from build123d import *

# Parameters (mm, degrees)
ESBO_O1_R                = 3.5
RESSALTO_EXTRUS_O1_DEPTH = 6
FILETE1_R                = 3
CHANFRO1_SIZE            = 2
CORTE_EXTRUS_O1_DEPTH    = 6
RESSALTO_EXTRUS_O2_DEPTH = 6
CORTE_EXTRUS_O2_DEPTH    = 10
FILETE2_R                = 2
CORTE_EXTRUS_O3_DEPTH    = 10
CORTE_EXTRUS_O4_DEPTH    = 201.089979759
CORTE_EXTRUS_O5_DEPTH    = 201.089979759
FILETE3_R                = 3


with BuildPart() as part:
    # Esboço1 → Ressalto-extrusão1 (new body)
    with BuildSketch(Plane.XY):
        with BuildLine():
            Line((23.094010768, 160), (88, 160))
            Line((88, 160), (100, 142.530265141))
            Line((100, 142.530265141), (100, 114))
            Line((100, 114), (84, 114))
            Line((84, 114), (69, 135.837168574))
            Line((69, 135.837168574), (69, 144))
            ThreePointArc((69, 144), (65, 148), (61, 144))
            Line((61, 144), (61, 135.837168574))
            Line((61, 135.837168574), (38, 96))
            Line((38, 96), (38, 0))
            Line((38, 0), (0, 0))
            Line((0, 0), (0, 120))
            Line((0, 120), (23.094010768, 160))
        make_face()
        with Locations((19, 12)):
            Circle(ESBO_O1_R, mode=Mode.SUBTRACT)
        with Locations((19, 24)):
            Circle(ESBO_O1_R, mode=Mode.SUBTRACT)
        with Locations((19, 36)):
            Circle(ESBO_O1_R, mode=Mode.SUBTRACT)
        with Locations((92, 122)):
            Circle(ESBO_O1_R, mode=Mode.SUBTRACT)
        with Locations((38, 122)):
            Circle(ESBO_O1_R, mode=Mode.SUBTRACT)
        with BuildLine():
            Line((41, 156), (49, 156))
            ThreePointArc((49, 156), (51, 154), (49, 152))
            Line((49, 152), (41, 152))
            ThreePointArc((41, 152), (39, 154), (41, 156))
        make_face(mode=Mode.SUBTRACT)
        with BuildLine():
            Line((8, 115), (8, 105))
            ThreePointArc((8, 105), (6, 103), (4, 105))
            Line((4, 105), (4, 115))
            ThreePointArc((4, 115), (6, 117), (8, 115))
        make_face(mode=Mode.SUBTRACT)
    extrude(amount=RESSALTO_EXTRUS_O1_DEPTH)

    # Filete1
    filete1_edges = [part.edges().sort_by_distance(p)[0] for p in [
        (100, 114, 3),
        (84, 114, 3),
        (69, 135.837168574, 3),
        (61, 135.837168574, 3),
        (38, 96, 3),
    ]]
    fillet(filete1_edges, radius=FILETE1_R)

    # Chanfro1
    chanfro1_edges = [part.edges().sort_by_distance(p)[0] for p in [
        (38, 0, 3),
        (0, 0, 3),
    ]]
    chamfer(chanfro1_edges, length=CHANFRO1_SIZE)

    # Esboço2 → Corte-extrusão1 (cut)
    with BuildSketch(Plane.XY.offset(6)):
        with BuildLine():
            Line((75, 152), (75, 141.231728845))
            Line((75, 141.231728845), (85.255212875, 126.30207469))
            ThreePointArc((85.255212875, 126.30207469), (88.154001919, 129.014862704), (92, 130))
            Line((92, 130), (92, 140.047327347))
            Line((92, 140.047327347), (83.789682385, 152))
            Line((83.789682385, 152), (75, 152))
        make_face()
        with BuildLine():
            Line((38, 130), (38, 140.047327347))
            Line((38, 140.047327347), (40.28207662, 144))
            Line((40.28207662, 144), (55, 144))
            Line((55, 144), (55, 141.444863729))
            Line((55, 141.444863729), (45.452626018, 124.908326913))
            ThreePointArc((45.452626018, 124.908326913), (42.512947191, 128.605551275), (38, 130))
        make_face()
    extrude(amount=-CORTE_EXTRUS_O1_DEPTH, mode=Mode.SUBTRACT)

    # Esboço3 → Ressalto-extrusão2 (add, through all)
    with BuildSketch(Plane.XY.offset(6)):
        Polygon((100, 142.530265141), (120, 113.414040375), (120, 77), (117, 74), (102.060706719, 74), (100, 77), (100, 90.707020188), (83.106053471, 115.301417403), (100, 117), align=None)
    extrude(amount=-RESSALTO_EXTRUS_O2_DEPTH)

    # Esboço4 → Corte-extrusão2 (cut)
    with BuildSketch(Plane.XY.offset(6)):
        with BuildLine():
            Line((105.122276139, 120.943770271), (114, 108.019480105))
            Line((114, 108.019480105), (114, 80))
            Line((114, 80), (106, 80))
            Line((106, 80), (106, 96.101580458))
            Line((106, 96.101580458), (93.595183818, 114.160651265))
            ThreePointArc((93.595183818, 114.160651265), (97.506753293, 116.196925973), (99.745062186, 119.996500127))
            ThreePointArc((99.745062186, 119.996500127), (102.128983719, 122.199693371), (105.122276139, 120.943770271))
        make_face()
    extrude(amount=-CORTE_EXTRUS_O2_DEPTH, mode=Mode.SUBTRACT)

    # Filete2
    filete2_edges = [part.edges().sort_by_distance(p)[0] for p in [
        (75, 152, 3),
        (92, 130, 3),
        (85.255212875, 126.30207469, 3),
        (45.452626018, 124.908326913, 3),
        (38, 130, 3),
        (38, 140.047327347, 3),
        (40.28207662, 144, 3),
        (55, 144, 3),
        (114, 108.019480105, 3),
        (114, 80, 3),
        (106, 80, 3),
        (106, 96.101580458, 3),
        (93.595183818, 114.160651265, 3),
    ]]
    fillet(filete2_edges, radius=FILETE2_R)

    # Esboço5 → Corte-extrusão3 (cut)
    with BuildSketch(Plane.XY.offset(6)):
        with BuildLine():
            ThreePointArc((19.000000124, 0), (11.718734325, 2.46149015), (7.424595906, 8.836138426))
            Line((7.424595906, 8.836138426), (0, 36))
            Line((0, 36), (0, 0))
            Line((0, 0), (19.000000124, 0))
        make_face()
        with BuildLine():
            ThreePointArc((30.575404094, 8.836138426), (26.281265774, 2.461490225), (19.000000124, 0))
            Line((19.000000124, 0), (38, 0))
            Line((38, 0), (38, 36))
            Line((38, 36), (30.575404094, 8.836138426))
        make_face()
        with BuildLine():
            Line((30, 65), (30, 41))
            ThreePointArc((30, 41), (29.707106781, 40.292893219), (29, 40))
            Line((29, 40), (28.124143795, 40))
            ThreePointArc((28.124143795, 40), (26.79716619, 40.309436781), (25.743932371, 41.173913043))
            ThreePointArc((25.743932371, 41.173913043), (19, 44.5), (12.256067629, 41.173913043))
            ThreePointArc((12.256067629, 41.173913043), (11.20283381, 40.309436781), (9.875856205, 40))
            Line((9.875856205, 40), (9, 40))
            ThreePointArc((9, 40), (8.292893219, 40.292893219), (8, 41))
            Line((8, 41), (8, 65))
            ThreePointArc((8, 65), (8.878679656, 67.121320344), (11, 68))
            Line((11, 68), (27, 68))
            ThreePointArc((27, 68), (29.121320344, 67.121320344), (30, 65))
        make_face()
        with BuildLine():
            ThreePointArc((30, 79), (29.121320344, 76.878679656), (27, 76))
            Line((27, 76), (11, 76))
            ThreePointArc((11, 76), (8.878679656, 76.878679656), (8, 79))
            Line((8, 79), (8, 88.08580312))
            Line((8, 88.08580312), (24.401923789, 116.494768463))
            ThreePointArc((24.401923789, 116.494768463), (27.776457135, 117.892545942), (30, 114.994768463))
            Line((30, 114.994768463), (30, 79))
        make_face()
    extrude(amount=-CORTE_EXTRUS_O3_DEPTH, mode=Mode.SUBTRACT)

    # Esboço6 → Corte-extrusão4 (cut, through all)
    with BuildSketch(Plane.XY.offset(6)):
        with BuildLine():
            Line((31, 156), (49, 156))
            ThreePointArc((49, 156), (51, 154), (49, 152))
            Line((49, 152), (31, 152))
            ThreePointArc((31, 152), (29, 154), (31, 156))
        make_face()
    extrude(amount=-CORTE_EXTRUS_O4_DEPTH, mode=Mode.SUBTRACT)

    # Esboço7 → Corte-extrusão5 (cut, through all)
    with BuildSketch(Plane.XY.offset(6)):
        with BuildLine():
            Line((23.094010768, 160), (9.770017724, 136.92216709))
            ThreePointArc((9.770017724, 136.92216709), (21.270577597, 145.667537692), (23.094010768, 160))
        make_face()
    extrude(amount=-CORTE_EXTRUS_O5_DEPTH, mode=Mode.SUBTRACT)

    # Filete3
    filete3_edges = [part.edges().sort_by_distance(p)[0] for p in [
        (23.094010768, 160, 3),
    ]]
    fillet(filete3_edges, radius=FILETE3_R)


solid = part.part
Design review of the part built by this model. Coordinates are the model's own, in mm. A direction names the side the tool comes from. Give positions to 0.01 mm unless a question says otherwise; leave off trailing zeros. Loops run counter-clockwise (first coordinate to the right, second up) from the corner with the lowest first, then second, coordinate; pieces in that order, holes last. Notation, with made-up numbers: (-21.75, 70.5) - (-1.75, 70.5) arc R19 ccw to (-1.75, 86.5) - close; hole circle Ø1 at (8.25, -38). An arc over 180 degrees is marked (long way). Write item = value, one per line.
1) Take a section at A-A on y = 24. State the section outline as (x, z) points, and give its area (3 significant figures).
Result sheet:
outline = (3.28, 0) - (15.5, 0) - (15.5, 6) - (3.28, 6) - close; (22.5, 0) - (34.72, 0) - (34.72, 6) - (22.5, 6) - close
area = 147 mm2
2) Take a section at C-C on z = 1.5. Count the separate pieces of the cut face and the enclosed holes in it, and give its area (3 significant figures).
Result sheet:
separate_pieces = 1
enclosed_holes = 12
area = 6,170 mm2
3) Take a section at B-B on x = 65. State the section outline as (y, z) points, and give its area (3 significant figures).
Result sheet:
outline = (148, 0) - (160, 0) - (160, 6) - (148, 6) - close
area = 72.0 mm2
4) Tool access review of faces 4 (the face through (110, 74, 3)), 5 (the face through (3.764, 22.228, 3.042)), 6 (the face through (19, 68, 3)): name each direction out of +Z, -Z, +X, -X, +Y, -Y from which nothing blocks a thin tool from reaching the whole face with its end or side.
Result sheet:
face_4 = +Z, -Z, +X, -Y
face_5 = +Z, -Z, -X, -Y
face_6 = +Z, -Z
5) Clearance check with flat-ended pins moving along their axes: pin 1 Ø6.5 at (x, y) = (19, 36) entering from +Z; pin 2 Ø3 at (y, z) = (53, 4) entering from +X; pin 3 Ø3 at (y, z) = (136, 1.5) entering from +X; pin 4 Ø1.5 at (x, z) = (57, 4.5) entering from -Y. State where each tip first meets the part, or that it passes through.
Result sheet:
pin_1 = through
pin_2 = 38
pin_3 = 105.52
pin_4 = 127.61
6) Draft analysis for pull direction Y (two halves, no side actions). For faces 1 (the face through (120, 95, 3)), 2 (the face through (47, 144, 3)), 3 (the face through (49.655, 116.188, 2.958)), state which applies: +Y half, -Y half, draft (parallel to the pull), parting line (faces both ways), or undercut.
Result sheet:
face_1 = draft
face_2 = undercut
face_3 = -Y half
7) To check wall thickness, follow line 1 (X direction, y = 128.5, z = 4); line 2 (X direction, y = 78, z = 2); line 3 (X direction, y = 146.5, z = 5.5). State the ranges of each line that lie inside material, in increasing order.
Result sheet:
line_1 = 4.91 to 42.66, 47.53 to 56.76, 74.04 to 83.75, 87.34 to 109.64
line_2 = 0 to 8.17, 29.83 to 38, 100 to 120
line_3 = 21.72 to 61.88, 68.12 to 75, 87.57 to 97.27
